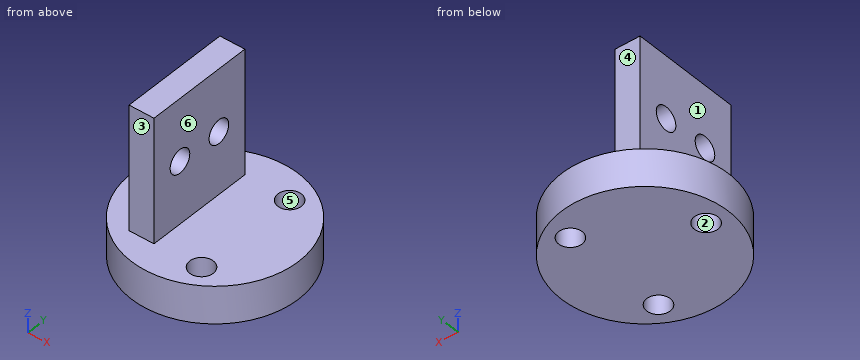
```python
from build123d import *

# Parameters (mm, degrees)
SKETCH2_R            = 8.509
BOSS_EXTRUDE1_DEPTH  = 3.81
SKETCH4_W            = 2.54
SKETCH4_H            = 11.1125
BOSS_EXTRUDE2_DEPTH  = 12.7
M2_CLEARANCE_HOLE1_D = 2.4
M2_CLEARANCE_HOLE2_D = 2.4


with BuildPart() as part:
    # Sketch2 → Boss-Extrude1 (new body)
    with BuildSketch(Plane.XY):
        Circle(SKETCH2_R)
    extrude(amount=BOSS_EXTRUDE1_DEPTH)

    # Sketch4 → Boss-Extrude2 (add)
    with BuildSketch(Plane.XY.offset(3.81)):
        with Locations((-2.8575, 0)):
            Rectangle(SKETCH4_W, SKETCH4_H)
    extrude(amount=BOSS_EXTRUDE2_DEPTH)

    # M2 Clearance Hole1 (through all)
    with Locations(Plane.XY.offset(3.81)):
        with Locations((-6.223, 0), (3.1115, 5.389276088), (3.1115, -5.389276088)):
            Hole(M2_CLEARANCE_HOLE1_D / 2)

    # M2 Clearance Hole2 (through all)
    with Locations(Plane(origin=(-1.5875, 0, 0), x_dir=(0, 0, -1), z_dir=(1, 0, 0))):
        with Locations((-10.16, -2.38125), (-10.16, 2.38125)):
            Hole(M2_CLEARANCE_HOLE2_D / 2)


solid = part.part
```
Here's how the part is built. I have some questions about the finished solid (model axes, mm). Face numbers are marked on the shaded views. A direction names the side the tool comes from. Round coordinates to 2 decimals unless told otherwise and drop trailing zeros. Loops run counter-clockwise (first coordinate to the right, second up) from the corner with the lowest first, then second, coordinate; pieces in that order, holes last.
1. Will these pins go through, and if not, where does the flat tip stop? pin 1 (3 mm diameter, centred on y = -2.38, z = 10.16, fed in from -X); pin 2 (1.9 mm diameter, centred on x = 3.11, y = 5.39, fed in from -Z); pin 3 (3 mm diameter, centred on x = -3.5, z = 13, fed in from -Y); pin 4 (6 mm diameter, centred on y = -5, z = 13.5, fed in from +X).
Answers:
pin 1: stops at x = -4.13
pin 2: passes through
pin 3: stops at y = -5.56
pin 4: stops at x = -1.59
2. Suppose I cut it at D-D, the plane z = 3.5. Please give me the cut outline in (x, y), and give its area (3 significant figures).
Answers:
outline: circle Ø17.02 at (0, 0); hole circle Ø2.4 at (-6.22, 0); hole circle Ø2.4 at (3.11, -5.39); hole circle Ø2.4 at (3.11, 5.39)
area: 214 mm2
3. Suppose I cut it at C-C, the plane x = -3.5. Please give me the cut outline in (y, z).
Answers:
outline: (-7.76, 0) - (7.76, 0) - (7.76, 3.81) - (5.56, 3.81) - (5.56, 16.51) - (-5.56, 16.51) - (-5.56, 3.81) - (-7.76, 3.81) - close; hole circle Ø2.4 at (-2.38, 10.16); hole circle Ø2.4 at (2.38, 10.16)
4. If I drill on probe 1 along Y at (x, z) = (-3.05, 10.16); probe 2 along Z at (x, y) = (-3.75, -2.5); probe 3 along Z at (x, y) = (0, -3.75), over which ranges is the centre line in solid material (lowest first)?
Answers:
probe 1: y = -5.56 to -3.58, -1.18 to 1.18, 3.58 to 5.56
probe 2: z = 0 to 8.97, 11.35 to 16.51
probe 3: z = 0 to 3.81
5. For the marked faces 4, 5 and 6, which set-ups out of +Z, -Z, +X, -X, +Y, -Y let a thin tool reach every point of the face, with its end or its side?
Answers:
face 4: +Z, +X, -X, +Y
face 5: +Z, -Z
face 6: +Z, +X, +Y, -Y
6. Suppose I cut it at B-B, the plane x = -6. Please give me the cut outline in (y, z), and give its area (3 significant figures).
Answers:
outline: (-6.03, 0) - (-1.18, 0) - (-1.18, 3.81) - (-6.03, 3.81) - close; (1.18, 0) - (6.03, 0) - (6.03, 3.81) - (1.18, 3.81) - close
area: 37.0 mm2
7. Suppose I cut it at A-A, the plane y = 0. Please give me the cut outline in (x, z), and give its area (3 significant figures).
Answers:
outline: (-8.51, 0) - (-7.42, 0) - (-7.42, 3.81) - (-8.51, 3.81) - close; (-5.02, 0) - (8.51, 0) - (8.51, 3.81) - (-1.59, 3.81) - (-1.59, 16.51) - (-4.13, 16.51) - (-4.13, 3.81) - (-5.02, 3.81) - close
area: 88.0 mm2
8. Thinking about a two-plate mould opening in X: for the marked faces 1, 2 and 3, which applies, released by +X, released by -X, zero draft, split by the parting line, or undercut?
Answers:
face 1: released by -X
face 2: undercut
face 3: zero draft
